Check sheet for the drawn part. Datum: minimum x, y, z corner. Units: mm. A direction names the side the tool comes from. Round coordinates to 2 decimals unless told otherwise and drop trailing zeros. Loops run counter-clockwise (first coordinate to the right, second up) from the corner with the lowest first, then second, coordinate; pieces in that order, holes last. Notation, with made-up numbers: (70.25, 51.25) -> (94.25, 51.25) arc R18 ccw to (94.25, 74.25) -> close; hole circle Ø3 at (62.25, 52.5). An arc over 180 degrees is marked (long way). Return JSON: item names as keys, results as strings.
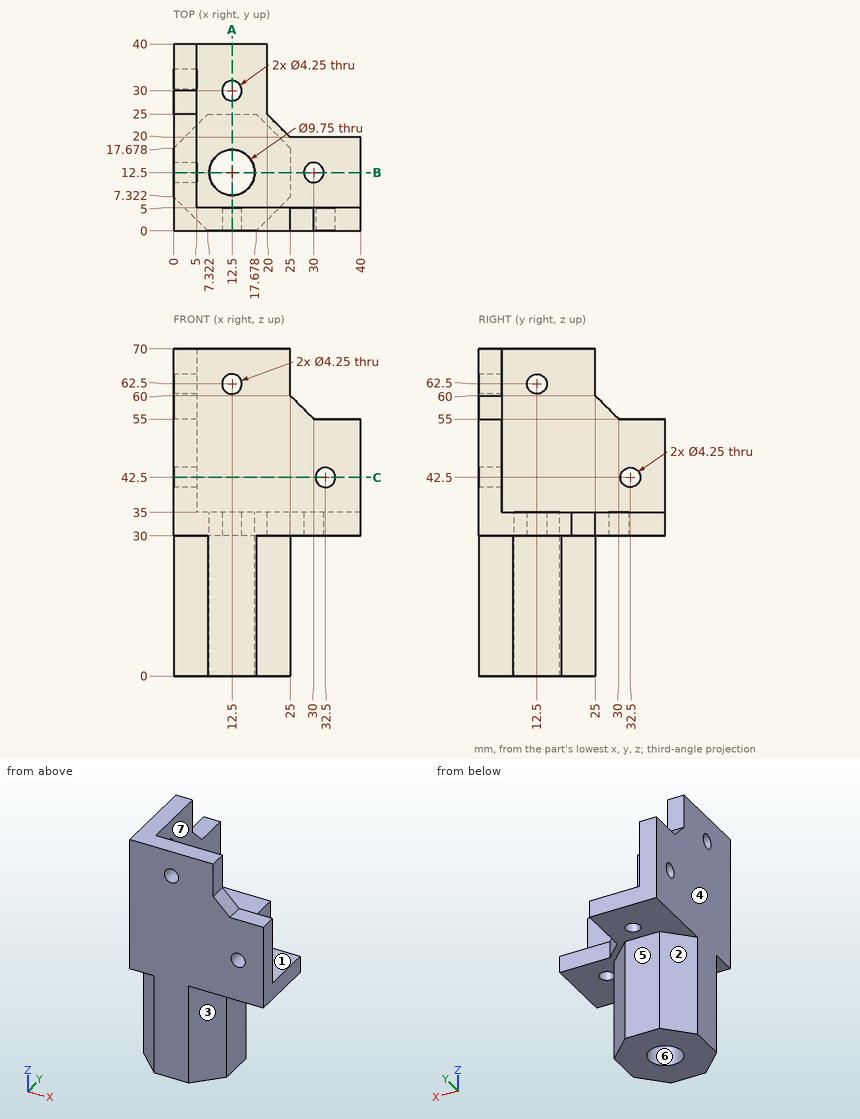
Q1. Draft check along X on the marked faces 4, 5, 6 and 7. Enter one of: released by +X, released by -X, zero draft, split by the parting line, or undercut.
Results list:
{"face 4": "released by -X", "face 5": "zero draft", "face 6": "undercut", "face 7": "released by +X"}
Q2. Tool access check on the marked faces 1, 2 and 3. Record the directions out of +Z, -Z, +X, -X, +Y, -Y that give a thin tool (end or side, any length) a straight path to the whole face; none if there is none.
Results list:
{"face 1": "+Z, +X, +Y", "face 2": "-Z, -X, +Y", "face 3": "-Z, +X, -Y"}
Q3. Section check C-C (z = 42.5). Record the boundary of the cut face in (x, y) (1 decimal).
Results list:
{"outline": "(0, 0) -> (30.4, 0) -> (30.4, 5) -> (5, 5) -> (5, 30.4) -> (0, 30.4) -> close; (0, 34.6) -> (5, 34.6) -> (5, 40) -> (0, 40) -> close; (34.6, 0) -> (40, 0) -> (40, 5) -> (34.6, 5) -> close"}
Q4. Material ranges on line 1 (Y direction, x = 12.5, z = 33.75) (1 decimal); line 2 (Z direction, x = 1.05, y = 12.5) (1 decimal); line 3 (X direction, y = 12.5, z = 17) (1 decimal), recorded low to high.
Results list:
{"line 1": "0 to 7.6, 17.4 to 27.9, 32.1 to 40", "line 2": "0 to 60.4, 64.6 to 70", "line 3": "0 to 7.6, 17.4 to 25"}
Q5. Section check A-A (x = 12.5). Record the boundary of the cut face in (y, z) (1 decimal).
Results list:
{"outline": "(0, 0) -> (7.6, 0) -> (7.6, 35) -> (5, 35) -> (5, 60.4) -> (0, 60.4) -> close; (0, 64.6) -> (5, 64.6) -> (5, 70) -> (0, 70) -> close; (17.4, 0) -> (25, 0) -> (25, 30) -> (27.9, 30) -> (27.9, 35) -> (17.4, 35) -> close; (32.1, 30) -> (40, 30) -> (40, 35) -> (32.1, 35) -> close"}
Q6. Go/stop test with flat-tipped pins: pin 1 (8 mm diameter, centred on x = 32.5, z = 29, fed in from +Y); pin 2 (10.5 mm diameter, centred on y = 16.5, z = 49, fed in from +X); pin 3 (5 mm diameter, centred on x = 10.5, z = 14.5, fed in from +Y). Record where each tip stops, or that it passes through.
Results list:
{"pin 1": "y = 20", "pin 2": "x = 5", "pin 3": "y = 25"}
